Design review of the part shown in the three views and the two pictorial views. Dimensions are in mm from the part's minimum x, y and z. A direction names the side the tool comes from. Coordinates: 2 decimals unless noted, no trailing zeros. Loops run counter-clockwise (first coordinate to the right, second up) from the corner with the lowest first, then second, coordinate; pieces in that order, holes last.
Q1. Add section D-D on y = 19. Give the boundary of the cut face in (x, z), and give its area (3 significant figures).
Q2. Machinability: for the marked faces 1 and 2, which of the approach directions +Z, -Z, +X, -X, +Y, -Y give a long, thin tool a straight path to every point of the face, cutting with its end or side? Answer none if there is none.
Q3. Wall thickness on probe 1 along Y at (x, z) = (11, 12.5); probe 2 along Z at (x, y) = (17.25, 4); probe 3 along Y at (x, z) = (4.5, 10.5): over which ranges is each line inside the solid? List them lowest first.
Q4. Add section A-A on y = 11. Give the boundary of the cut face in (x, z).
Q5. Add section C-C on z = 11.5. Give the boundary of the cut face in (x, y).
Q6. Draft analysis for pull direction X (two halves, no side actions). For the marked faces 3, 4, 5 and 6, state which applies: released by +X, released by -X, zero draft, split by the parting line, or undercut.
Q7. For P1, Ø2, axis at x = 15.5, y = 16.5, coming from the +Z side; P2, Ø10, axis at x = 4, y = 19, coming from the -Z side; P3, Ø8, axis at x = 16.5, z = 3.5, coming from the -Y side, all flat-tipped, find the tip position at first contact; note any pin that passes through.
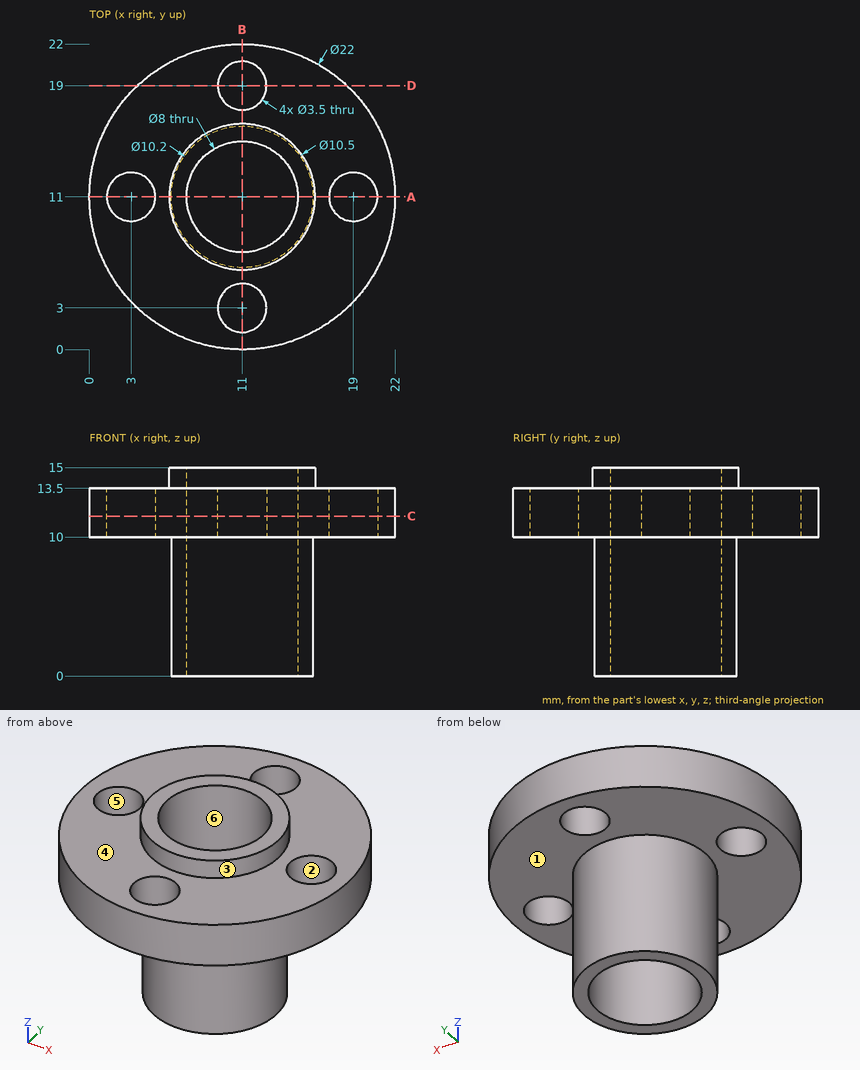
Entries:
1. outline: (3.45, 10) - (9.25, 10) - (9.25, 13.5) - (3.45, 13.5) - close; (12.75, 10) - (18.55, 10) - (18.55, 13.5) - (12.75, 13.5) - close
1. area: 40.6 mm2
2. face 1: -Z
2. face 2: +Z, -Z
3. probe 1: y = 0 to 1.25, 4.75 to 7, 15 to 17.25, 20.75 to 22
3. probe 2: z = 10 to 13.5
3. probe 3: y = 2.13 to 10.1, 11.9 to 19.87
4. outline: (0, 10) - (1.25, 10) - (1.25, 13.5) - (0, 13.5) - close; (4.75, 10) - (5.9, 10) - (5.9, 0) - (7, 0) - (7, 15) - (5.75, 15) - (5.75, 13.5) - (4.75, 13.5) - close; (15, 0) - (16.1, 0) - (16.1, 10) - (17.25, 10) - (17.25, 13.5) - (16.25, 13.5) - (16.25, 15) - (15, 15) - close; (20.75, 10) - (22, 10) - (22, 13.5) - (20.75, 13.5) - close
5. outline: circle Ø22 at (11, 11); hole circle Ø3.5 at (3, 11); hole circle Ø8 at (11, 11); hole circle Ø3.5 at (11, 3); hole circle Ø3.5 at (11, 19); hole circle Ø3.5 at (19, 11)
6. face 3: split by the parting line
6. face 4: zero draft
6. face 5: undercut
6. face 6: undercut
7. P1: stops at z = 13.5
7. P2: stops at z = 10
7. P3: stops at y = 6.13
